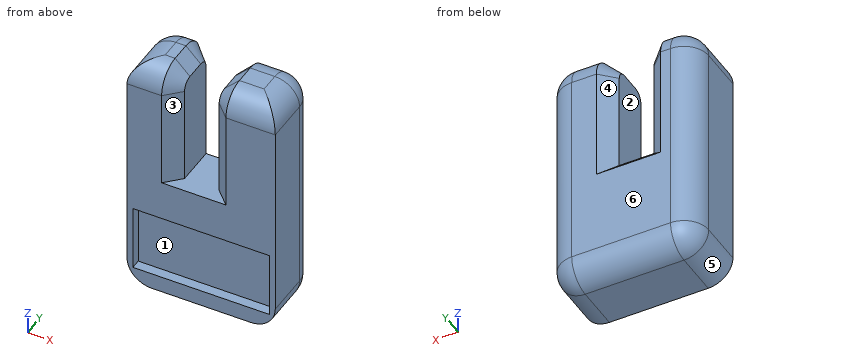
```python
from build123d import *

# Parameters (mm, degrees)
F0_W     = 27.7
F0_H     = 13.5
F1_DEPTH = 14
F2_R     = 5
F4_W     = 27.7
F4_H     = 13.5
F5_DEPTH = 2
F6_SIZE  = 3


with BuildPart() as f1:
    # F0 (on Front) → F1 (new body)
    with BuildSketch(Plane.XZ):
        Polygon((-13.2842407189, 29.1734449556), (-13.2842407189, -20.8265550444), (16.7157592811, -20.8265550444), (16.7157592811, 29.1734449556), (3.7307592811, 29.1734449556), (3.7307592811, 4.1734449556), (-3.2842407189, 4.1734449556), (-3.2842407189, 29.1734449556), align=None)
        with Locations((1.7157592811, -10.8674009684)):
            Rectangle(F0_W, F0_H, mode=Mode.SUBTRACT)
        with Locations((1.7157592811, -10.8674009684)):
            Rectangle(F0_W, F0_H)
    extrude(amount=F1_DEPTH)

    # F2
    f2_edges = [f1.edges().sort_by_distance(p)[0] for p in [
        (1.715759, 0, -20.826555),
        (-13.284241, 0, 4.173445),
        (16.715759, 0, 4.173445),
        (16.715759, -7, -20.826555),
        (-13.284241, -7, -20.826555),
        (-8.284241, 0, 29.173445),
        (10.223259, 0, 29.173445),
        (-13.284241, -7, 29.173445),
        (16.715759, -7, 29.173445),
        (10.223259, -14, 29.173445),
        (-8.284241, -14, 29.173445),
    ]]
    fillet(f2_edges, radius=F2_R)

    # F4 (on face) → F5 (cut)
    with BuildSketch(Plane.XZ.offset(14)):
        with Locations((1.7414525137, -10.761866346)):
            Rectangle(F4_W, F4_H)
    extrude(amount=-F5_DEPTH, mode=Mode.SUBTRACT)

    # F6
    f6_edges = [f1.edges().sort_by_distance(p)[0] for p in [
        (-3.284241, 0, 14.173445),
        (3.730759, 0, 14.173445),
        (0.223259, 0, 4.173445),
    ]]
    chamfer(f6_edges, length=F6_SIZE)


solid = f1.part
```
Geometry: final body of the model. Coordinates: model frame, mm. Face numbers are marked on the shaded views. A direction names the side the tool comes from. Coordinates: 2 decimals unless noted, no trailing zeros. Write each loop counter-clockwise with the first axis right and the second up, starting at its lowest first coordinate (ties: lowest second). Pieces come first, ordered by that corner, then holes. Notation, with made-up numbers: M 37.25,-2 L 44.25,-2 A13 cw 44.25,21 Z; hole C 67.25,46.5 d8. An arc over 180 degrees is marked long. Use CSV: the item, a comma, the result in double quotes. Start each with the question number.
1. Cut plane C-C on z = -12. Return the cut outline in (x, y).
2. Cut plane D-D on y = -8.25. Return the cut outline in (x, z).
3. Cut plane B-B on x = -2.5. Return the cut outline in (y, z).
4. First-contact query: P1, Ø2, axis at y = -3, z = 19.5, coming from the -X side; P2, Ø1.6, axis at x = -4, y = -13.5, coming from the +Z side; P3, Ø5.5, axis at x = 1.5, y = -8, coming from the +Z side. Flat tips, straight axial feed; report the tip coordinate or a pass-through.
5. Mould query, pull axis X, two halves, no side actions, for the marked faces 4, 5 and 6. Classes: pulls with the +X half, pulls with the -X half, needs draft (parallel to the pull), parting line crosses it, or undercut.
6. Reachability of the marked faces 1, 2 and 3 from +Z, -Z, +X, -X, +Y, -Y: full face, straight path, thin tool, end or side. Return the list, or none.
7. Ray query, probe 1 along X at (y, z) = (-7, 19); probe 2 along Z at (x, y) = (-2.5, -11.5); probe 3 along Z at (x, y) = (-3, -12.5). Return the intervals inside material, ascending.
8. Cut plane A-A on z = 19.5. Return the cut outline in (x, y).
Entries:
1,outline,"M -13.28,-14 L -12.11,-14 L -12.11,-12 L 15.59,-12 L 15.59,-14 L 16.72,-14 L 16.72,-5 A5 ccw 11.72,0 L -8.28,0 A5 ccw -13.28,-5 Z"
2,outline,"M -13.28,-15.83 A5 ccw -8.28,-20.83 L 11.72,-20.83 A5 ccw 16.72,-15.83 L 16.72,24.17 A5 ccw 11.72,29.17 L 6.73,29.17 L 3.73,26.17 L 3.73,4.17 L -3.28,4.17 L -3.28,26.17 L -6.28,29.17 L -8.28,29.17 A5 ccw -13.28,24.17 Z"
3,outline,"M -14,-20.83 L -5,-20.83 A5 ccw 0,-15.83 L 0,1.17 L -3,4.17 L -14,4.17 L -14,-4.01 L -12,-4.01 L -12,-17.51 L -14,-17.51 Z"
4,P1,"x = -13.18"
4,P2,"z = 4.17"
4,P3,"z = 26.69"
5,face 4,"undercut"
5,face 5,"pulls with the -X half"
5,face 6,"needs draft"
6,face 1,"-Y"
6,face 2,"+Z, +Y, -Y"
6,face 3,"+Z, -Y"
7,probe 1,"-13.28 to -3.28, 3.73 to 16.72"
7,probe 2,"-20.83 to 4.17"
7,probe 3,"-20.83 to -17.51, -4.01 to 4.17"
8,outline,"M -13.28,-14 L -6.28,-14 L -3.28,-11 L -3.28,-3 L -6.28,0 L -8.28,0 A5 ccw -13.28,-5 Z; M 3.73,-11 L 6.73,-14 L 16.72,-14 L 16.72,-5 A5 ccw 11.72,0 L 6.73,0 L 3.73,-3 Z"
